from build123d import *


with BuildPart() as part:
    # Croquis1 → Revolución1 (revolve)
    with BuildSketch(Plane.XY):
        with BuildLine():
            Line((9.858, 26), (13.4, 26))
            ThreePointArc((13.4, 26), (13.824264069, 26.175735931), (14, 26.6))
            Line((14, 26.6), (14, 34.4))
            ThreePointArc((14, 34.4), (13.824264069, 34.824264069), (13.4, 35))
            Line((13.4, 35), (9.858, 35))
            Line((9.858, 35), (9.858, 32.142666563))
            ThreePointArc((9.858, 32.142666563), (10.572, 30), (9.858, 27.857333437))
            Line((9.858, 27.857333437), (9.858, 26))
        make_face()
    revolve(axis=Axis((13.4, 0, 0), (-1, 0, 0)))


solid = part.part
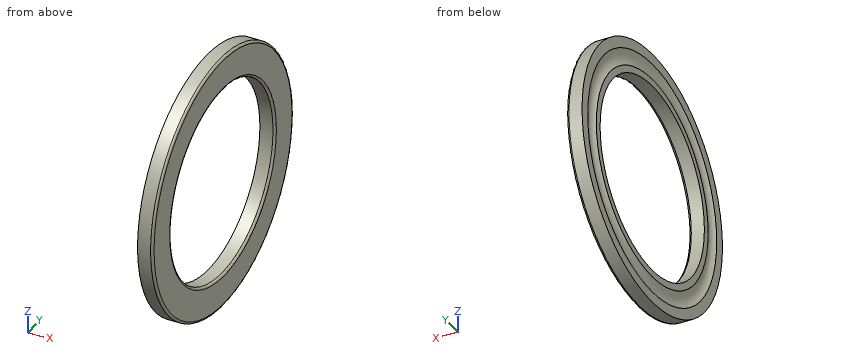
Model file for the job. Use its own axes, mm. Give positions to 0.01 mm unless a question says otherwise; leave off trailing zeros. Order: outer loops, then holes, each group sorted by start corner. A loop starts at its lowest first (then second) coordinate and runs counter-clockwise, first axis right, second up. Notation, with made-up numbers: M 18.5,-9.5 L 68.5,-9.5 A10 cw 68.5,-3.5 Z; hole C -15.5,12.25 d10. An arc over 180 degrees is marked long. Write item = value, one per line.
Q1. Cut at A-A, the plane y = 0. List the corners of the cut face in (x, z), then the cut area to 3 significant figures.
Derived:
outline = M 9.86,-35 L 13.4,-35 A0.6 ccw 14,-34.4 L 14,-26.6 A0.6 ccw 13.4,-26 L 9.86,-26 L 9.86,-27.86 A3.57 cw 9.86,-32.14 Z; M 9.86,26 L 13.4,26 A0.6 ccw 14,26.6 L 14,34.4 A0.6 ccw 13.4,35 L 9.86,35 L 9.86,32.14 A3.57 cw 9.86,27.86 Z
area = 70.1 mm2
Q2. Drill centre lines: line 1 (Z direction, x = 12.1, y = 0); line 2 (Y direction, x = 13.8, z = -21.5). Where is each one in solid material? Low to high. Write a range as [from, to].
Derived:
line_1 = [-35, -26], [26, 35]
line_2 = [-27.42, -14.89], [14.89, 27.42]
Q3. Flat gauge pin, fed straight in: pin 1 (2 mm diameter, centred on x = 10.5, y = 1.5, fed in from -Z). Where does the tip first touch, or does it go through?
Derived:
pin_1 = -35
Q4. Cut at C-C, the plane x = 11.5. List the corners of the cut face in (y, z), then the cut area to 3 significant figures.
Derived:
outline = C 0,0 d70; hole C 0,0 d52
area = 1,720 mm2
